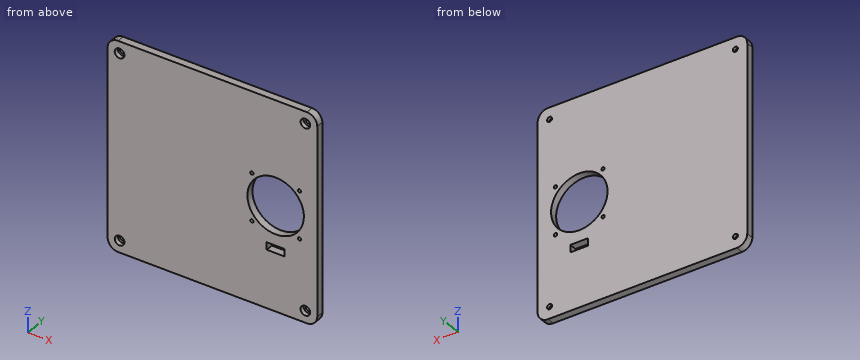
from build123d import *

# Parameters (mm, degrees)
SKETCH1_W                      = 141
SKETCH1_H                      = 141
BOSS_EXTRUDE1_DEPTH            = 5
CUT_EXTRUDE1_REACH             = 101.827
SKETCH3_R                      = 1.1
CBORE_FOR_M3_SHCS1_D           = 3.4
CBORE_FOR_M3_SHCS1_CBORE_D     = 6.5
CBORE_FOR_M3_SHCS1_CBORE_DEPTH = 3
FILLET1_R                      = 7
ESQUISSE1_R                    = 19
ENL_V_MAT_EXTRU_1_DEPTH        = 100.827350962
ESQUISSE2_W                    = 12
ESQUISSE2_H                    = 5
ENL_V_MAT_EXTRU_2_DEPTH        = 100.827350962


with BuildPart() as part:
    # Sketch1 → Boss-Extrude1 (new body)
    with BuildSketch(Plane(origin=(0, 0, 0), x_dir=(1, 0, 0), z_dir=(0, 1, 0))):
        Rectangle(SKETCH1_W, SKETCH1_H)
    extrude(amount=BOSS_EXTRUDE1_DEPTH)

    # Sketch3 → Cut-Extrude1 (cut, up to next)
    with BuildSketch(Plane(origin=(0, 5, 0), x_dir=(1, 0, 0), z_dir=(0, 1, 0)), mode=Mode.PRIVATE) as cut_extrude1_sk1:
        with Locations(Location((26.5, 16, 0), (0, 0, 270))):
            Circle(SKETCH3_R)
    cut_extrude1_tool1 = extrude(cut_extrude1_sk1.sketch, amount=-CUT_EXTRUDE1_REACH, mode=Mode.PRIVATE) & part.part
    # Sketch3 → Cut-Extrude1 (cut, up to next)
    with BuildSketch(Plane(origin=(0, 5, 0), x_dir=(1, 0, 0), z_dir=(0, 1, 0)), mode=Mode.PRIVATE) as cut_extrude1_sk2:
        with Locations(Location((58.5, 16, 0), (0, 0, 270))):
            Circle(SKETCH3_R)
    cut_extrude1_tool2 = extrude(cut_extrude1_sk2.sketch, amount=-CUT_EXTRUDE1_REACH, mode=Mode.PRIVATE) & part.part
    # Sketch3 → Cut-Extrude1 (cut, up to next)
    with BuildSketch(Plane(origin=(0, 5, 0), x_dir=(1, 0, 0), z_dir=(0, 1, 0)), mode=Mode.PRIVATE) as cut_extrude1_sk3:
        with Locations(Location((58.5, -16, 0), (0, 0, 270))):
            Circle(SKETCH3_R)
    cut_extrude1_tool3 = extrude(cut_extrude1_sk3.sketch, amount=-CUT_EXTRUDE1_REACH, mode=Mode.PRIVATE) & part.part
    # Sketch3 → Cut-Extrude1 (cut, up to next)
    with BuildSketch(Plane(origin=(0, 5, 0), x_dir=(1, 0, 0), z_dir=(0, 1, 0)), mode=Mode.PRIVATE) as cut_extrude1_sk4:
        with Locations(Location((26.5, -16, 0), (0, 0, 270))):
            Circle(SKETCH3_R)
    cut_extrude1_tool4 = extrude(cut_extrude1_sk4.sketch, amount=-CUT_EXTRUDE1_REACH, mode=Mode.PRIVATE) & part.part
    add(cut_extrude1_tool1.solids().sort_by_distance((26.5, 5, -16))[0], mode=Mode.SUBTRACT)
    add(cut_extrude1_tool2.solids().sort_by_distance((58.5, 5, -16))[0], mode=Mode.SUBTRACT)
    add(cut_extrude1_tool3.solids().sort_by_distance((58.5, 5, 16))[0], mode=Mode.SUBTRACT)
    add(cut_extrude1_tool4.solids().sort_by_distance((26.5, 5, 16))[0], mode=Mode.SUBTRACT)

    # CBORE for M3 SHCS1 (through all)
    with Locations(Plane(origin=(-62.5, 0, 62.5), x_dir=(0, 0, -1), z_dir=(0, -1, 0))):
        with Locations((0, 0), (125, 0), (125, 125), (0, 125)):
            CounterBoreHole(CBORE_FOR_M3_SHCS1_D / 2, CBORE_FOR_M3_SHCS1_CBORE_D / 2, CBORE_FOR_M3_SHCS1_CBORE_DEPTH)

    # Fillet1
    fillet1_edges = [part.edges().sort_by_distance(p)[0] for p in [
        (70.5, 2.5, 70.5),
        (-70.5, 2.5, 70.5),
        (-70.5, 2.5, -70.5),
        (70.5, 2.5, -70.5),
    ]]
    fillet(fillet1_edges, radius=FILLET1_R)

    # Esquisse1 → Enlèv. mat.-Extru.1 (cut, through all)
    with BuildSketch(Plane.XZ):
        with Locations(Location((42.5, 0, 0), (0, 0, 270))):
            Circle(ESQUISSE1_R)
    extrude(amount=-ENL_V_MAT_EXTRU_1_DEPTH, mode=Mode.SUBTRACT)

    # Esquisse2 → Enlèv. mat.-Extru.2 (cut, through all)
    with BuildSketch(Plane.XZ):
        with Locations((42.5, -29)):
            Rectangle(ESQUISSE2_W, ESQUISSE2_H)
    extrude(amount=-ENL_V_MAT_EXTRU_2_DEPTH, mode=Mode.SUBTRACT)


solid = part.part
Geometry check sheet. Reference: the model listing, model coordinates, mm. Give positions to 0.01 mm unless a question says otherwise; leave off trailing zeros. Loops run counter-clockwise (first coordinate to the right, second up) from the corner with the lowest first, then second, coordinate; pieces in that order, holes last. Notation, with made-up numbers: M 80,89 L 115,89 A20 ccw 115,100 Z; hole C 43.5,27 d3. An arc over 180 degrees is marked long. Write each question's results on one line, items separated by ' | '.
1) Section check B-B, the plane z = 0. Record the boundary of the cut face in (x, y).
Answers follow:
outline: M -70.5,0 L 23.5,0 L 23.5,5 L -70.5,5 Z; M 61.5,0 L 70.5,0 L 70.5,5 L 61.5,5 Z
2) Section check A-A, the plane y = 0.9. Count the separate pieces of the cut face and the enclosed holes in it, plus the area to 3 significant figures.
Answers follow:
separate pieces: 1 | enclosed holes: 10 | area: 18,500 mm2
3) Section check C-C, the plane x = 34. Record the boundary of the cut face in (y, z).
Answers follow:
outline: M 0,-70.5 L 5,-70.5 L 5,-16.99 L 0,-16.99 Z; M 0,16.99 L 5,16.99 L 5,70.5 L 0,70.5 Z
4) Thickness scan on line 1 (X direction, y = 1.4, z = -62.5); line 2 (X direction, y = 4.3, z = 62.5); line 3 (X direction, y = 1.75, z = -16). Record the ranges inside material, lowest first.
Answers follow:
line 1: -70.5 to -65.75, -59.25 to 59.25, 65.75 to 70.5 | line 2: -70.5 to -64.2, -60.8 to 60.8, 64.2 to 70.5 | line 3: -70.5 to 25.4, 27.6 to 32.25, 52.75 to 57.4, 59.6 to 70.5
5) Gauge pin test, flat end, axial feed: pin 1 (5 mm diameter, centred on x = -63, z = 62.5, fed in from -Y). Record the tip position at first contact, or that the pin passes through.
Answers follow:
pin 1: y = 3
